from build123d import *

# Parameters (mm, degrees)
PAD_DEPTH    = 15
FILLET_R     = 5
FILLET001_R  = 2
FILLET002_R  = 1
FILLET003_R  = 1
PAD001_DEPTH = 8


with BuildPart() as part:
    # Sketch → Pad (new body)
    with BuildSketch(Plane.XY):
        Polygon((0, 0), (0, 75), (100, 75), (100, 78), (103, 78), (103, 55), (45, 55), (10, 20), (10, 0), align=None)
        Polygon((18.660254, 55), (18.660254, 60), (14.330127, 62.5), (10, 60), (10, 55), (14.330127, 52.5), align=None, mode=Mode.SUBTRACT)
        Polygon((24.490381, 44.901924), (24.490381, 49.901924), (20.160254, 52.401924), (15.830127, 49.901924), (15.830127, 44.901924), (20.160254, 42.401924), align=None, mode=Mode.SUBTRACT)
        Polygon((30.320508, 55), (30.320508, 60), (25.990381, 62.5), (21.660254, 60), (21.660254, 55), (25.990381, 52.5), align=None, mode=Mode.SUBTRACT)
    extrude(amount=PAD_DEPTH)

    # Fillet
    fillet_edges = [part.edges().sort_by_distance(p)[0] for p in [
        (50, 75, 15),
        (50, 75, 0),
    ]]
    fillet(fillet_edges, radius=FILLET_R)

    # Fillet001
    fillet001_edges = [part.edges().sort_by_distance(p)[0] for p in [
        (101.5, 78, 15),
        (101.5, 78, 0),
    ]]
    fillet(fillet001_edges, radius=FILLET001_R)

    # Fillet002
    fillet002_edges = [part.edges().sort_by_distance(p)[0] for p in [
        (10, 10, 15),
        (27.5, 37.5, 15),
        (27.5, 37.5, 0),
        (10, 10, 0),
        (74, 55, 15),
        (74, 55, 0),
        (103, 55, 7.5),
        (5, 0, 15),
        (5, 0, 0),
        (10, 0, 7.5),
        (103, 65.5, 15),
        (103, 65.5, 0),
        (103, 78, 7.5),
        (103, 77.414214, 14.414214),
        (103, 77.414214, 0.585786),
    ]]
    fillet(fillet002_edges, radius=FILLET002_R)

    # Fillet003
    fillet003_edges = [part.edges().sort_by_distance(p)[0] for p in [
        (100, 73.535534, 13.535534),
        (100, 75, 7.5),
        (100, 73.535534, 1.464466),
    ]]
    fillet(fillet003_edges, radius=FILLET003_R)

    # Sketch003 → Pad001 (join)
    with BuildSketch(Plane.XY):
        Polygon((0, 60.8), (-3.3, 60.8), (-3.3, 59), (-2.5, 59), (-2.5, 60), (0, 60), align=None)
        Polygon((0, 55), (0, 55.8), (-3.3, 55.8), (-3.3, 54), (-2.5, 54), (-2.5, 55), align=None)
        Polygon((0, 50.8), (-3.3, 50.8), (-3.3, 49), (-2.5, 49), (-2.5, 50), (0, 50), align=None)
        Polygon((0, 25.8), (-3.3, 25.8), (-3.3, 24), (-2.5, 24), (-2.5, 25), (0, 25), align=None)
        Polygon((0, 20.8), (-3.3, 20.8), (-3.3, 19), (-2.5, 19), (-2.5, 20), (0, 20), align=None)
        Polygon((0, 15.8), (-3.3, 15.8), (-3.3, 14), (-2.5, 14), (-2.5, 15), (0, 15), align=None)
    extrude(amount=PAD001_DEPTH)


solid = part.part
Work out the finished part from the listing and answer in its coordinate system (mm). A direction names the side the tool comes from. Round coordinates to 2 decimals unless told otherwise and drop trailing zeros. Loops run counter-clockwise (first coordinate to the right, second up) from the corner with the lowest first, then second, coordinate; pieces in that order, holes last. Notation, with made-up numbers: (-3.75, -10) - (34.25, -10) arc R30 ccw to (34.25, 15) - close; hole circle Ø2 at (-3, 43). An arc over 180 degrees is marked (long way). One line per item, written item: value.
Q1. Find section B-B on z = 3.5. State how many separate pieces and enclosed holes the cut face has, and give its area (3 significant figures).
Check values:
separate pieces: 1
enclosed holes: 3
area: 3,030 mm2
Q2. Straight lines are drawn through the part: probe 1 along Y at (x, z) = (95, 6.5); probe 2 along Y at (x, z) = (11, 2.75); probe 3 along Y at (x, z) = (20.5, 3.5). For each, find the intervals that lie inside material, in ascending order.
Check values:
probe 1: 55 to 75
probe 2: 21 to 54.42, 60.58 to 74.47
probe 3: 30.5 to 42.6, 52.21 to 74.77
Q3. Each of these flat-tipped pins is pushed along its axis until it touches: pin 1 Ø4 at (y, z) = (46.5, 5) entering from -X; pin 2 Ø8 at (x, z) = (40, 5) entering from -Y; pin 3 Ø0.6 at (x, z) = (-3, 2.5) entering from -Y. Where does it stop, or does it pass through?
Check values:
pin 1: x = 0
pin 2: y = 46
pin 3: y = 14
Q4. Find section A-A on x = 57. Give the vertices of the cut face in (y, z), and give its area (3 significant figures).
Check values:
outline: (55, 1) arc R1 ccw to (56, 0) - (70, 0) arc R5 ccw to (75, 5) - (75, 10) arc R5 ccw to (70, 15) - (56, 15) arc R1 ccw to (55, 14) - close
area: 289 mm2
Q5. The mould has two halves that part along X. Classify faces 1 (the flat face through (-1, 15, 4)), 2 (the flat face through (-2, 15.8, 4)), 3 (the cylindrical face through (27.04, 37.46, 0.29)): +X half, -X half, draft (parallel to the pull), parting line (faces both ways), or undercut.
Check values:
face 1: undercut
face 2: draft
face 3: +X half
Q6. For faces 4 (the flat face through (-2, 55.8, 4)), 5 (the cylindrical face through (50, 74, 2)), 6 (the flat face through (28.125, 53.732, 7.395)), determine the directions among +Z, -Z, +X, -X, +Y, -Y from which every point of the face is accessible in a straight line to the end or side of a thin tool.
Check values:
face 4: +Z, -Z, -X
face 5: -Z, -X, +Y
face 6: +Z, -Z
